Could you check a few things on this model? Use its own coordinates, in mm. A direction names the side the tool comes from. Round coordinates to 2 decimals unless told otherwise and drop trailing zeros. Loops run counter-clockwise (first coordinate to the right, second up) from the corner with the lowest first, then second, coordinate; pieces in that order, holes last. Notation, with made-up numbers: (41, 18.25) -> (96, 18.25) arc R19 ccw to (96, 29.25) -> close; hole circle Ø4 at (26.5, 25.25). An arc over 180 degrees is marked (long way). Use CSV: the item, a comma, the result in double quotes. Start each with the question number.
```python
from build123d import *

# Parameters (mm, degrees)
F0_R         = 1.25
F0_R_2       = 5.25
F1_DEPTH     = 2
F2_DEPTH     = 20
F3_DEPTH     = 20
F4_T4_DEPTH  = 68.3486393209
F4_S5_R      = 21
F4_T6_DEPTH  = 36
F4_T10_DEPTH = 68.3486393209
F4_S11_R     = 21
F4_T12_DEPTH = 36
F5_T2_ANGLE  = 272.1691776214
F6_R         = 1.5
F7_DEPTH     = 25
F6_R_2       = 3
F8_DEPTH     = 16
F10_DEPTH    = 11


# Not quite as in the source:
# - a fillet or chamfer that OpenCascade refuses, or shapes differently, is made with other operations: its cross-section is extruded or revolved along the edge and cut away or added


with BuildPart() as f1:
    # F0 (on Top) → F1 (new body)
    with BuildSketch(Plane.XY):
        Polygon((-9.3097730907, -16.125), (9.3097730907, -16.125), (18.6195461814, 0), (9.3097730907, 16.125), (-9.3097730907, 16.125), (-18.6195461814, 0), align=None)
        with Locations((6.982329818, -12.09375)):
            Circle(F0_R, mode=Mode.SUBTRACT)
        with Locations((-13.964659636, 0)):
            Circle(F0_R, mode=Mode.SUBTRACT)
        Circle(F0_R_2, mode=Mode.SUBTRACT)
        with Locations((6.982329818, 12.09375)):
            Circle(F0_R, mode=Mode.SUBTRACT)
    extrude(amount=F1_DEPTH)

    # F0 (on Top) → F2 (join)
    with BuildSketch(Plane.XY):
        with BuildLine():
            ThreePointArc((-10.5, 18.1865334795), (-10.5, -18.1865334795), (21, 0))
            ThreePointArc((21, 0), (10.5, 18.1865334795), (-10.5, 18.1865334795))
        make_face()
        Polygon((18.6195461814, 0), (9.3097730907, -16.125), (-9.3097730907, -16.125), (-18.6195461814, 0), (-9.3097730907, 16.125), (9.3097730907, 16.125), align=None, mode=Mode.SUBTRACT)
    extrude(amount=F2_DEPTH)

    # F0 (on Top) → F3 (join)
    with BuildSketch(Plane.XY):
        with BuildLine():
            ThreePointArc((-10.5, 18.1865334795), (10.5, 18.1865334795), (21, 0))
            Line((21, 0), (28, 0))
            ThreePointArc((28, 0), (14, 24.248711306), (-14, 24.248711306))
            Line((-14, 24.248711306), (-10.5, 18.1865334795))
        make_face()
    extrude(amount=F3_DEPTH)

    # F4: chamfer of 7 on 2 edges, made by hand


with BuildPart() as f4_tool2:
    # F4_s3 → F4_t4 (new body)
    with BuildSketch(Plane.XY.offset(-24.1743196605)):
        with BuildLine():
            Line((-9.8994949366, 17.1464281995), (-5.1164228135, 27.5285709326))
            ThreePointArc((-5.1164228135, 27.5285709326), (-9.6039256501, 26.3014184429), (-14, 24.248711306))
            Line((-14, 24.248711306), (-9.8994949366, 17.1464281995))
        make_face()
    extrude(amount=F4_T4_DEPTH)

    # F4_s5 → F4_t6 (cut, symmetric)
    with BuildSketch(Plane.XY.offset(10)):
        Circle(F4_S5_R)
    extrude(amount=F4_T6_DEPTH, both=True, mode=Mode.SUBTRACT)


with BuildPart() as f1_1:
    add(f1.part)

    # F4_t1: cut F4_tool2
    add(f4_tool2.part, mode=Mode.SUBTRACT)


with BuildPart() as f4_tool8:
    # F4_s9 → F4_t10 (new body)
    with BuildSketch(Plane.XY.offset(-24.1743196605)):
        with BuildLine():
            Line((19.7989898732, 0), (26.3986531643, 9.3333333333))
            ThreePointArc((26.3986531643, 9.3333333333), (27.5796593521, 4.8334656324), (28, 0))
            Line((28, 0), (19.7989898732, 0))
        make_face()
    extrude(amount=F4_T10_DEPTH)

    # F4_s11 → F4_t12 (cut, symmetric)
    with BuildSketch(Plane.XY.offset(10)):
        Circle(F4_S11_R)
    extrude(amount=F4_T12_DEPTH, both=True, mode=Mode.SUBTRACT)


with BuildPart() as f1_2:
    add(f1_1.part)

    # F4_t7: cut F4_tool8
    add(f4_tool8.part, mode=Mode.SUBTRACT)

    # F5: chamfer of 18 x 7 on 1 edges, made by hand

    # F5_s1 → F5_t2 (revolve, cut)
    with BuildSketch(Plane(origin=(0, 0, 0), x_dir=(0, 0, 1), z_dir=(-0.9706518309, -0.2404891332, 0))):
        Polygon((18, -28), (0, -21), (0, -28), align=None)
    revolve(axis=Axis((0, 0, 0), (0, 0, 1)), revolution_arc=F5_T2_ANGLE, mode=Mode.SUBTRACT)

    # F6 (on face) → F7 (cut)
    with BuildSketch(Plane.XY):
        with Locations((21.8586163831, 10.5006375909)):
            Circle(F6_R)
        with Locations((-2.3912845495, 24.1318100897)):
            Circle(F6_R)
    extrude(amount=F7_DEPTH, mode=Mode.SUBTRACT)

    # F6 (on face) → F8 (cut)
    with BuildSketch(Plane.XY):
        with Locations((-2.3912845495, 24.1318100897)):
            Circle(F6_R_2)
        with Locations((-2.3912845495, 24.1318100897)):
            Circle(F6_R, mode=Mode.SUBTRACT)
        with Locations((21.8586163831, 10.5006375909)):
            Circle(F6_R_2)
        with Locations((21.8586163831, 10.5006375909)):
            Circle(F6_R, mode=Mode.SUBTRACT)
    extrude(amount=F8_DEPTH, mode=Mode.SUBTRACT)

    # F9 (on face) → F10 (cut)
    with BuildSketch(Plane.XY.offset(20)):
        with BuildLine():
            ThreePointArc((16.6565165694, -3.4000670246), (16.9139111633, -1.7086863843), (17, 0))
            ThreePointArc((17, 0), (16.9139111633, 1.7086863843), (16.6565165694, 3.4000670246))
            Line((16.6565165694, 3.4000670246), (11.2728027026, 12.7249329754))
            ThreePointArc((11.2728027026, 12.7249329754), (8.5, 14.7224318643), (5.3837138668, 16.125))
            Line((5.3837138668, 16.125), (-5.3837138668, 16.125))
            ThreePointArc((-5.3837138668, 16.125), (-8.5, 14.7224318643), (-11.2728027026, 12.7249329754))
            Line((-11.2728027026, 12.7249329754), (-16.6565165694, 3.4000670246))
            ThreePointArc((-16.6565165694, 3.4000670246), (-17, 0), (-16.6565165694, -3.4000670246))
            Line((-16.6565165694, -3.4000670246), (-11.2728027026, -12.7249329754))
            ThreePointArc((-11.2728027026, -12.7249329754), (-8.5, -14.7224318643), (-5.3837138668, -16.125))
            Line((-5.3837138668, -16.125), (5.3837138668, -16.125))
            ThreePointArc((5.3837138668, -16.125), (8.5, -14.7224318643), (11.2728027026, -12.7249329754))
            Line((11.2728027026, -12.7249329754), (16.6565165694, -3.4000670246))
        make_face()
        with BuildLine():
            Line((11.2728027026, 12.7249329754), (16.6565165694, 3.4000670246))
            ThreePointArc((16.6565165694, 3.4000670246), (14.7224318643, 8.5), (11.2728027026, 12.7249329754))
        make_face()
        with BuildLine():
            ThreePointArc((11.2728027026, -12.7249329754), (14.7224318643, -8.5), (16.6565165694, -3.4000670246))
            Line((16.6565165694, -3.4000670246), (11.2728027026, -12.7249329754))
        make_face()
        with BuildLine():
            Line((-5.3837138668, 16.125), (5.3837138668, 16.125))
            ThreePointArc((5.3837138668, 16.125), (0, 17), (-5.3837138668, 16.125))
        make_face()
        with BuildLine():
            ThreePointArc((-5.3837138668, -16.125), (0, -17), (5.3837138668, -16.125))
            Line((5.3837138668, -16.125), (-5.3837138668, -16.125))
        make_face()
        with BuildLine():
            Line((-16.6565165694, 3.4000670246), (-11.2728027026, 12.7249329754))
            ThreePointArc((-11.2728027026, 12.7249329754), (-14.7224318643, 8.5), (-16.6565165694, 3.4000670246))
        make_face()
        with BuildLine():
            ThreePointArc((-16.6565165694, -3.4000670246), (-14.7224318643, -8.5), (-11.2728027026, -12.7249329754))
            Line((-11.2728027026, -12.7249329754), (-16.6565165694, -3.4000670246))
        make_face()
    extrude(amount=-F10_DEPTH, mode=Mode.SUBTRACT)


solid = f1_2.part
```
1. Suppose I cut it at B-B (z = 3.5). List the corners of the cut face in (x, y) for me (3 decimals), then the cut area to 3 significant figures.
2. Suppose I cut it at A-A (x = 0). List the corners of the cut face in (y, z) for me (3 decimals), then the cut area to 3 significant figures.
3. Will these pins go through, and if not, where does the flat tip stop? pin 1 (6 mm diameter, centred on x = 2, z = 4.5, fed in from -Y); pin 2 (4 mm diameter, centred on x = -13.5, z = 16.5, fed in from -Y); pin 3 (2 mm diameter, centred on x = -14.5, z = 15.5, fed in from -Y).
4. For faces 4 (the face through (7.65, 13.15, 0.99)), 5 (the face through (-15, -8, 15)), 6 (the face through (-2, 26, 16)), which set-ups out of +Z, -Z, +X, -X, +Y, -Y let a thin tool reach every point of the face, with its end or its side?
5. If I drill on L1, parallel to Z at x = -6, y = 10; L2, parallel to X at y = -4.5, z = 4.5; L3, parallel to X at y = -13, z = 12.75, over which ranges is the centre line in solid material (lowest first)?
6. Suppose I cut it at C-C (x = -14). List the corners of the cut face in (y, z) for me.
7. We'd pull the mould along X, two halves only. Please class faces 1 (the face through (6.1, 16.3, 20)), 2 (the face through (-14.4, -8.4, 9)), 3 (the face through (14, 8, 7)): pulls with the +X half, pulls with the -X half, needs draft (parallel to the pull), parting line crosses it, or undercut.
Geometry check:
1,outline,"(-9.074, 18.938) arc R21 ccw (long way) to (20.938, 1.611) -> (22.119, 3.281) arc R22.361 ccw to (21.023, 7.619) arc R3 cw to (19.087, 11.649) arc R22.361 ccw to (0.03, 22.361) arc R3 cw to (-4.418, 21.92) arc R22.361 ccw to (-8.218, 20.796) -> close; hole (-18.62, 0) -> (-9.31, -16.125) -> (9.31, -16.125) -> (18.62, 0) -> (9.31, 16.125) -> (-9.31, 16.125) -> close"
1,area,"533 mm²"
2,outline,"(-21, 0) -> (-5.25, 0) -> (-5.25, 2) -> (-16.125, 2) -> (-16.125, 9) -> (-17, 9) -> (-17, 20) -> (-21, 20) -> close; (5.25, 0) -> (21, 0) -> (22.32, 3.395) -> (22.32, 16) -> (25.943, 16) -> (25.943, 12.712) -> (28, 18) -> (28, 20) -> (17, 20) -> (17, 9) -> (16.125, 9) -> (16.125, 2) -> (5.25, 2) -> close"
2,area,"267 mm²"
3,pin 1,"stops at y = -21"
3,pin 2,"stops at y = -17.57"
3,pin 3,"stops at y = -16.09"
4,face 4,"+Z, -Z"
4,face 5,"+Z"
4,face 6,"-Z"
5,L1,"z = 0 to 2"
5,L2,"x = -20.51 to -16.02, 16.02 to 20.51"
5,L3,"x = -16.49 to -11.11, 11.11 to 16.49"
6,outline,"(-15.65, 0) -> (-1.25, 0) -> (-1.25, 2) -> (-8, 2) -> (-8, 9) -> (-9.64, 9) -> (-9.64, 20) -> (-15.65, 20) -> close; (1.25, 0) -> (15.65, 0) -> (15.65, 20) -> (9.64, 20) -> (9.64, 9) -> (8, 9) -> (8, 2) -> (1.25, 2) -> close"
7,face 1,"needs draft"
7,face 2,"undercut"
7,face 3,"undercut"
